Model file for the job. Use its own axes, mm. Face numbers are marked on the shaded views. A direction names the side the tool comes from. Give positions to 0.01 mm unless a question says otherwise; leave off trailing zeros. Loops run counter-clockwise (first coordinate to the right, second up) from the corner with the lowest first, then second, coordinate; pieces in that order, holes last. Notation, with made-up numbers: (22, -20.75) - (73, -20.75) arc R30 ccw to (73, 8.25) - close; hole circle Ø2 at (-7, 68). An arc over 180 degrees is marked (long way). Use a Markdown table: item, result.
from build123d import *

# Parameters (mm, degrees)
F0_W     = 384.175
F0_H     = 609.6
F1_DEPTH = 914.4
F2_T     = -12.7
F3_W     = 28.575
F3_H     = 17.4625
F3_W_2   = 301.625
F3_W_3   = 4.7625
F3_H_2   = 6.35
F4_DEPTH = 19.05
F5_DEPTH = 19.05
F3_H_3   = 395.2875
F3_W_4   = 254
F3_H_4   = 333.375
F6_DEPTH = 19.05
F7_W     = 7.9375
F7_H     = 333.375
F8_DEPTH = 254


with BuildPart() as f1:
    # F0 (on Top) → F1 (new body)
    with BuildSketch(Plane.XY):
        Rectangle(F0_W, F0_H)
    extrude(amount=F1_DEPTH)

    # F2
    f2_openings = [f1.faces().sort_by_distance(p)[0] for p in [
        (0, -304.8, 457.2),
    ]]
    offset(amount=F2_T, openings=f2_openings)

    # F3 (on face) → F4 (join)
    with BuildSketch(Plane.XZ.offset(304.8)):
        Polygon((-192.0875, 477.8375), (-192.0875, 436.5625), (-184.15, 436.5625), (-184.15, 454.025), (-179.3875, 454.025), (-179.3875, 460.375), (-184.15, 460.375), (-184.15, 477.8375), align=None)
        with Locations((-165.1, 445.29375)):
            Rectangle(F3_W, F3_H)
        with Locations((-165.1, 469.10625)):
            Rectangle(F3_W, F3_H)
        with Locations((0, 445.29375)):
            Rectangle(F3_W_2, F3_H)
        with Locations((0, 469.10625)):
            Rectangle(F3_W_2, F3_H)
        with Locations((165.1, 445.29375)):
            Rectangle(F3_W, F3_H)
        with Locations((165.1, 469.10625)):
            Rectangle(F3_W, F3_H)
        Polygon((184.15, 436.5625), (192.0875, 436.5625), (192.0875, 477.8375), (184.15, 477.8375), (184.15, 460.375), (179.3875, 460.375), (179.3875, 454.025), (184.15, 454.025), align=None)
        with Locations((181.76875, 445.29375)):
            Rectangle(F3_W_3, F3_H)
        with Locations((181.76875, 469.10625)):
            Rectangle(F3_W_3, F3_H)
        with Locations((165.1, 457.2)):
            Rectangle(F3_W, F3_H_2)
        with Locations((-165.1, 457.2)):
            Rectangle(F3_W, F3_H_2)
        with Locations((-181.76875, 445.29375)):
            Rectangle(F3_W_3, F3_H)
        with Locations((-181.76875, 469.10625)):
            Rectangle(F3_W_3, F3_H)
        with Locations((0, 457.2)):
            Rectangle(F3_W_2, F3_H_2)
    extrude(amount=-F4_DEPTH)

    # F3 (on face) → F5 (join)
    with BuildSketch(Plane.XZ.offset(304.8)):
        Polygon((-179.3875, 901.7), (-179.3875, 477.8375), (-150.8125, 477.8375), (-150.8125, 873.125), (150.8125, 873.125), (150.8125, 477.8375), (179.3875, 477.8375), (179.3875, 901.7), align=None)
        Polygon((-192.0875, 914.4), (-192.0875, 477.8375), (-184.15, 477.8375), (-184.15, 908.05), (184.15, 908.05), (184.15, 477.8375), (192.0875, 477.8375), (192.0875, 914.4), align=None)
        Polygon((-150.8125, 436.5625), (-179.3875, 436.5625), (-179.3875, 12.7), (179.3875, 12.7), (179.3875, 436.5625), (150.8125, 436.5625), (150.8125, 41.275), (-150.8125, 41.275), align=None)
        Polygon((-184.15, 436.5625), (-192.0875, 436.5625), (-192.0875, 0), (192.0875, 0), (192.0875, 436.5625), (184.15, 436.5625), (184.15, 6.35), (-184.15, 6.35), align=None)
        Polygon((-179.3875, 436.5625), (-184.15, 436.5625), (-184.15, 6.35), (184.15, 6.35), (184.15, 436.5625), (179.3875, 436.5625), (179.3875, 12.7), (-179.3875, 12.7), align=None)
        with Locations((-165.1, 445.29375)):
            Rectangle(F3_W, F3_H)
        Polygon((-192.0875, 477.8375), (-192.0875, 436.5625), (-184.15, 436.5625), (-184.15, 454.025), (-179.3875, 454.025), (-179.3875, 460.375), (-184.15, 460.375), (-184.15, 477.8375), align=None)
        with Locations((-181.76875, 445.29375)):
            Rectangle(F3_W_3, F3_H)
        with Locations((-165.1, 469.10625)):
            Rectangle(F3_W, F3_H)
        with Locations((165.1, 469.10625)):
            Rectangle(F3_W, F3_H)
        with Locations((165.1, 445.29375)):
            Rectangle(F3_W, F3_H)
        Polygon((184.15, 436.5625), (192.0875, 436.5625), (192.0875, 477.8375), (184.15, 477.8375), (184.15, 460.375), (179.3875, 460.375), (179.3875, 454.025), (184.15, 454.025), align=None)
        with Locations((181.76875, 445.29375)):
            Rectangle(F3_W_3, F3_H)
    extrude(amount=-F5_DEPTH)

    # F3 (on face) → F6 (join)
    with BuildSketch(Plane.XZ.offset(304.8)):
        Polygon((-150.8125, 436.5625), (-179.3875, 436.5625), (-179.3875, 12.7), (179.3875, 12.7), (179.3875, 436.5625), (150.8125, 436.5625), (150.8125, 41.275), (-150.8125, 41.275), align=None)
        Polygon((-179.3875, 436.5625), (-184.15, 436.5625), (-184.15, 6.35), (184.15, 6.35), (184.15, 436.5625), (179.3875, 436.5625), (179.3875, 12.7), (-179.3875, 12.7), align=None)
        with Locations((0, 238.91875)):
            Rectangle(F3_W_2, F3_H_3)
        with Locations((0, 230.1875)):
            Rectangle(F3_W_4, F3_H_4, mode=Mode.SUBTRACT)
        with Locations((0, 445.29375)):
            Rectangle(F3_W_2, F3_H)
        with Locations((-165.1, 445.29375)):
            Rectangle(F3_W, F3_H)
        with Locations((165.1, 445.29375)):
            Rectangle(F3_W, F3_H)
        with Locations((181.76875, 445.29375)):
            Rectangle(F3_W_3, F3_H)
        with Locations((-181.76875, 445.29375)):
            Rectangle(F3_W_3, F3_H)
        Polygon((-179.3875, 901.7), (-179.3875, 477.8375), (-150.8125, 477.8375), (-150.8125, 873.125), (150.8125, 873.125), (150.8125, 477.8375), (179.3875, 477.8375), (179.3875, 901.7), align=None)
        with Locations((0, 675.48125)):
            Rectangle(F3_W_2, F3_H_3)
        with Locations((0, 684.2125)):
            Rectangle(F3_W_4, F3_H_4, mode=Mode.SUBTRACT)
        with Locations((-165.1, 469.10625)):
            Rectangle(F3_W, F3_H)
        with Locations((0, 469.10625)):
            Rectangle(F3_W_2, F3_H)
        with Locations((165.1, 469.10625)):
            Rectangle(F3_W, F3_H)
        with Locations((181.76875, 469.10625)):
            Rectangle(F3_W_3, F3_H)
        Polygon((-184.15, 908.05), (-184.15, 477.8375), (-179.3875, 477.8375), (-179.3875, 901.7), (179.3875, 901.7), (179.3875, 477.8375), (184.15, 477.8375), (184.15, 908.05), align=None)
        with Locations((-181.76875, 469.10625)):
            Rectangle(F3_W_3, F3_H)
    extrude(amount=F6_DEPTH)

    # F7 (on face) → F8 (join, through all)
    with BuildSketch(Plane(origin=(127, 0, 0), x_dir=(0, -1, 0), z_dir=(-1, 0, 0))):
        with Locations((313.53125, 230.1875)):
            Rectangle(F7_W, F7_H)
        with Locations((313.53125, 684.2125)):
            Rectangle(F7_W, F7_H)
    extrude(amount=F8_DEPTH)


solid = f1.part
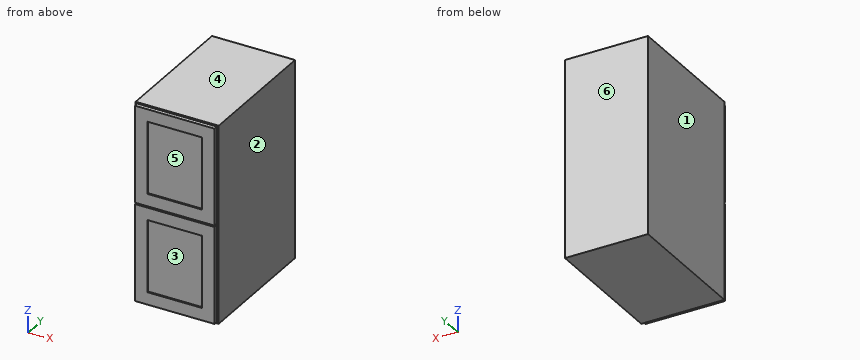
(1) Mould opens along X. For the marked faces 1, 2, 3 and 4 say: pulls with the +X half, pulls with the -X half, needs draft (parallel to the pull), parting line crosses it, or undercut.
Computed:
| item | result |
|---|---|
| face 1 | pulls with the -X half |
| face 2 | pulls with the +X half |
| face 3 | undercut |
| face 4 | needs draft |
(2) Slice it at C-C, the plane z = 343. Write the cut outline in (x, y).
Computed:
| item | result |
|---|---|
| outline | (-192.09, -304.8) - (-184.15, -304.8) - (-184.15, -323.85) - (-127, -323.85) - (-127, -317.5) - (127, -317.5) - (127, -323.85) - (184.15, -323.85) - (184.15, -304.8) - (192.09, -304.8) - (192.09, 304.8) - (-192.09, 304.8) - close; hole (-179.39, -285.75) - (-150.81, -285.75) - (-150.81, -304.8) - (-127, -304.8) - (-127, -309.56) - (127, -309.56) - (127, -304.8) - (150.81, -304.8) - (150.81, -285.75) - (179.39, -285.75) - (179.39, 292.1) - (-179.39, 292.1) - close |
(3) Slice it at A-A, the plane y = 213.5. Write the cut outline in (x, z).
Computed:
| item | result |
|---|---|
| outline | (-192.09, 0) - (192.09, 0) - (192.09, 914.4) - (-192.09, 914.4) - close; hole (-179.39, 12.7) - (179.39, 12.7) - (179.39, 901.7) - (-179.39, 901.7) - close |
(4) Slice it at B-B, the plane x = -161.5. Write the cut outline in (y, z) (3 decimals).
Computed:
| item | result |
|---|---|
| outline | (-323.85, 6.35) - (-304.8, 6.35) - (-304.8, 0) - (304.8, 0) - (304.8, 914.4) - (-304.8, 914.4) - (-304.8, 908.05) - (-323.85, 908.05) - (-323.85, 460.375) - (-304.8, 460.375) - (-304.8, 454.025) - (-323.85, 454.025) - close; hole (-285.75, 12.7) - (292.1, 12.7) - (292.1, 901.7) - (-285.75, 901.7) - close |
(5) 3-axis set-ups, long thin cutter, end or side, ignore diameter. For the marked faces 5 and 6: which of +Z, -Z, +X, -X, +Y, -Y reach the whole face in a straight line?
Computed:
| item | result |
|---|---|
| face 5 | -Y |
| face 6 | +Z, -Z, +X, -X, +Y |
(6) Pin check, flat tips, straight feed: P1, Ø5, axis at x = 51.5, y = -320.5, coming from the -Z side; P2, Ø5, axis at x = -1.5, y = -307.5, coming from the +Z side; P3, Ø4, axis at y = -306.5, z = 259, coming from the -X side; P4, Ø15, axis at y = -317, z = 198, coming from the -X side. Stop position of each tip, or through.
Computed:
| item | result |
|---|---|
| P1 | z = 6.35 |
| P2 | z = 908.05 |
| P3 | x = -192.09 |
| P4 | x = -184.15 |
(7) Drill centre lines: probe 1 along Z at (x, y) = (-16, -77); probe 2 along Y at (x, z) = (-108, 303); probe 3 along X at (y, z) = (120.5, 410). Where is each one in solid material? Low to high. Write a range as [from, to].
Computed:
| item | result |
|---|---|
| probe 1 | [0, 12.7], [901.7, 914.4] |
| probe 2 | [-317.5, -309.56], [292.1, 304.8] |
| probe 3 | [-192.09, -179.39], [179.39, 192.09] |
